Source: CAD feature listing. Evaluate the final solid. Frame: model axes, mm. A direction names the side the tool comes from. Give positions to 0.01 mm unless a question says otherwise; leave off trailing zeros. Order: outer loops, then holes, each group sorted by start corner. A loop starts at its lowest first (then second) coordinate and runs counter-clockwise, first axis right, second up. Notation, with made-up numbers: (42, 17.25) - (53, 17.25) arc R27 cw to (53, 37.25) - close; hole circle Ø7 at (9.25, 8.5). An arc over 180 degrees is marked (long way). Write each question's results on one line, items separated by ' | '. Start each with the question number.
Item 1: Section D-D on y = 0.85. Output: boundary loops of the cut face in (x, z) (3 decimals).
Item 2: Line query: line 1 along Z through (x, y) = (3, 1.9); line 2 along Z through (x, y) = (-2.25, 1); line 3 along Z through (x, y) = (0.75, 3.65). Output: solid intervals per line, ascending.
Item 3: Section C-C on z = 3. Output: boundary loops of the cut face in (x, y) (3 decimals).
Item 4: Section A-A on x = -2. Output: boundary loops of the cut face in (y, z), and give its area (3 significant figures).
Item 5: Set-up query: faces 1 (the flat face through (-7.85, 3, -18)), 2 (the flat face through (0, 3, -5.9)), 3 (the flat face through (0, 3, 5.9)), 4 (the flat face through (7.85, 3, -18)), 5 (the flat face through (-7, 3, 0)). Return all of +Z, -Z, +X, -X, +Y, -Y with unobstructed straight access to the full face (end or side cutting, diameter ignored); none if empty.
Item 6: Section B-B on y = 3.05. Output: boundary loops of the cut face in (x, z), and give its area (3 significant figures).
Item 7: Mould query, pull axis Z, two halves, no side actions, for faces 6 (the flat face through (0, 4.19, -18)), 7 (the flat face through (0, 1.65, 7)), 8 (the flat face through (0, 1, -15.4)). Classes: released by +Z, released by -Z, zero draft, split by the parting line, or undercut.
Item 8: Contact query for flat-ended pins moving along their axis: pin 1 Ø2 at (y, z) = (2.5, -18) entering from -X; pin 2 Ø2 at (x, z) = (-2.5, -20.5) entering from -Y; pin 3 Ø1 at (y, z) = (3, -2) entering from +X. Output: stop coordinate, or through.
Autodesk Inventor part; units mm, degrees
ref_plane "YZ Plane" through (0, 0, 0) normal (1, 0, 0) x (0, 1, 0)
ref_plane "XZ Plane" through (0, 0, 0) normal (0, 1, 0) x (-1, 0, 0)
ref_plane "XY Plane" through (0, 0, 0) normal (0, 0, 1) x (1, 0, 0)
sketch "Skizze1" plane through (0, 0, 0) normal (0, 1, 0) x (-1, 0, 0)
  line L0 (-8.975, 15.4) -> (8.975, 15.4)
  line L1 (8.975, 15.4) -> (8.975, -15.4)
  line L2 (8.975, -15.4) -> (-8.975, -15.4)
  line L3 (-8.975, -15.4) -> (-8.975, 15.4)
  line L4 (-8.975, 15.4) -> (8.975, -15.4) construction
  line L5 (8.975, 15.4) -> (-8.975, -15.4) construction
  point P0 (0, 0)
  dimension "d0" = 17.95
  dimension "d1" = 30.8
extrude "Extrusion1" add sketch "Skizze1" along normal blind 1.65
sketch "Skizze2" plane through (0, 1.65, 0) normal (0, 1, 0) x (1, 0, 0)
  line L0 (-7, 5.9) -> (7, 5.9)
  line L1 (7, 5.9) -> (7, -5.9)
  line L2 (7, -5.9) -> (-7, -5.9)
  line L3 (-7, -5.9) -> (-7, 5.9)
  line L4 (-7, 5.9) -> (7, -5.9) construction
  line L5 (7, 5.9) -> (-7, -5.9) construction
  point P0 (0, 0)
  dimension "d4" = 14
  dimension "d5" = 11.8
extrude "Extrusion2" add sketch "Skizze2" along normal blind 1.9
sketch "Skizze3" plane through (0, 1.65, 0) normal (0, 1, 0) x (1, 0, 0)
  line L0 (7, 5.9) -> (7, -5.9)
  line L1 (7, -5.9) -> (-7, -5.9)
  line L2 (-7, -5.9) -> (-7, 5.9)
  line L3 (-7, 5.9) -> (7, 5.9)
  line L4 (-8.975, -15.4) -> (8.975, -15.4)
  line L5 (8.975, -15.4) -> (8.975, 15.4)
  line L6 (8.975, 15.4) -> (-8.975, 15.4)
  line L7 (-8.975, 15.4) -> (-8.975, -15.4)
  line L8 (7.85, 12.45) -> (-7.85, 12.45)
  line L9 (-7.85, 12.45) -> (-7.85, 22.8)
  line L10 (-7.85, 22.8) -> (7.85, 22.8)
  line L11 (7.85, 22.8) -> (7.85, 12.45)
  line L12 (0, -0.0027) -> (0, 15.4) construction
  point P0 (0, 0)
  dimension "d8" = 15.7
  dimension "d9" = 2.95
  dimension "d10" = 38.2
  dimension "d11" = 10.35
extrude "Extrusion3" add sketch "Skizze3" along normal blind 2.54 contours L9 L10 L11 L6 | L6 L11 L8 L9
properties part number "FTDI_Friend"
Evaluation:
1) outline: (-8.975, -15.4) - (8.975, -15.4) - (8.975, 15.4) - (-8.975, 15.4) - close
2) line 1: z = -22.8 to -12.45, -5.9 to 5.9 | line 2: z = -15.4 to 15.4 | line 3: z = -22.8 to -12.45
3) outline: (-8.975, 0) - (8.975, 0) - (8.975, 1.65) - (7, 1.65) - (7, 3.55) - (-7, 3.55) - (-7, 1.65) - (-8.975, 1.65) - close
4) outline: (0, -15.4) - (1.65, -15.4) - (1.65, -22.8) - (4.19, -22.8) - (4.19, -12.45) - (1.65, -12.45) - (1.65, -5.9) - (3.55, -5.9) - (3.55, 5.9) - (1.65, 5.9) - (1.65, 15.4) - (0, 15.4) - close | area: 99.5 mm^2
5) face 1: +Z, -Z, -X, +Y | face 2: +X, -X, +Y | face 3: +Z, +X, -X, +Y | face 4: +Z, -Z, +X, +Y | face 5: +Z, -X, +Y
6) outline: (-7.85, -22.8) - (7.85, -22.8) - (7.85, -12.45) - (-7.85, -12.45) - close; (-7, -5.9) - (7, -5.9) - (7, 5.9) - (-7, 5.9) - close | area: 328 mm^2
7) face 6: zero draft | face 7: undercut | face 8: released by -Z
8) pin 1: stops at x = -7.85 | pin 2: stops at y = 1.65 | pin 3: stops at x = 7
